```python
from build123d import *

# Parameters (mm, degrees)
ESBO_O1_W                = 6.6
ESBO_O1_H                = 2.5
RESSALTO_EXTRUS_O1_DEPTH = 20
ESBO_O2_R                = 1.5
CORTE_EXTRUS_O1_DEPTH    = 26
ESBO_O4_R                = 1.8
CORTE_EXTRUS_O2_DEPTH    = 16


with BuildPart() as part:
    # Esboço1 → Ressalto-extrusão1 (new body)
    with BuildSketch(Plane.XY):
        with BuildLine():
            Line((-12, 0), (-12, -7))
            Line((-12, -7), (-21, -7))
            Line((-21, -7), (-21, -10))
            Line((-21, -10), (54, -10))
            Line((54, -10), (54, -7))
            Line((54, -7), (45, -7))
            Line((45, -7), (45, 0))
            ThreePointArc((45, 0), (43.507140429, 5.796550698), (39.4, 10.150862032))
            ThreePointArc((39.4, 10.150862032), (38.373214893, 11.239439866), (38, 12.68857754))
            Line((38, 12.68857754), (38, 15.080826084))
            Line((38, 15.080826084), (28, 15.080826084))
            Line((28, 15.080826084), (28, 12.68857754))
            ThreePointArc((28, 12.68857754), (27.626785107, 11.239439866), (26.6, 10.150862032))
            ThreePointArc((26.6, 10.150862032), (22.492859571, 5.796550698), (21, 0))
            Line((21, 0), (21, -7))
            Line((21, -7), (12, -7))
            Line((12, -7), (12, 0))
            ThreePointArc((12, 0), (10.507140429, 5.796550698), (6.4, 10.150862032))
            ThreePointArc((6.4, 10.150862032), (5.373214893, 11.239439866), (5, 12.68857754))
            Line((5, 12.68857754), (5, 15.080826084))
            Line((5, 15.080826084), (-5, 15.080826084))
            Line((-5, 15.080826084), (-5, 12.68857754))
            ThreePointArc((-5, 12.68857754), (-5.373214893, 11.239439866), (-6.4, 10.150862032))
            ThreePointArc((-6.4, 10.150862032), (-10.507140429, 5.796550698), (-12, 0))
        make_face()
        with Locations((0, 10.080826084)):
            Rectangle(ESBO_O1_W, ESBO_O1_H, mode=Mode.SUBTRACT)
        with Locations((33, 10.080826084)):
            Rectangle(ESBO_O1_W, ESBO_O1_H, mode=Mode.SUBTRACT)
        with BuildLine():
            ThreePointArc((7.8, 0), (0, 7.8), (-7.8, 0))
            ThreePointArc((-7.8, 0), (0, -7.8), (7.8, 0))
        make_face(mode=Mode.SUBTRACT)
        with BuildLine():
            ThreePointArc((40.8, 0), (33, -7.8), (25.2, 0))
            ThreePointArc((25.2, 0), (33, 7.8), (40.8, 0))
        make_face(mode=Mode.SUBTRACT)
    extrude(amount=RESSALTO_EXTRUS_O1_DEPTH)

    # Esboço2 → Corte-extrusão1 (cut)
    with BuildSketch(Plane(origin=(0, -7, 0), x_dir=(1, 0, 0), z_dir=(0, 1, 0))):
        with Locations((-16.5, -4)):
            Circle(ESBO_O2_R)
        with Locations((-16.5, -16)):
            Circle(ESBO_O2_R)
        with Locations((49.5, -16)):
            Circle(ESBO_O2_R)
        with Locations((49.5, -4)):
            Circle(ESBO_O2_R)
        with Locations((16.5, -10)):
            Circle(ESBO_O2_R)
    extrude(amount=-CORTE_EXTRUS_O1_DEPTH, mode=Mode.SUBTRACT)

    # Esboço4 → Corte-extrusão2 (cut)
    with BuildSketch(Plane(origin=(0, 15.080826084, 0), x_dir=(1, 0, 0), z_dir=(0, 1, 0))):
        with Locations((0, -10)):
            Circle(ESBO_O4_R)
        with Locations((33, -10)):
            Circle(ESBO_O4_R)
    extrude(amount=-CORTE_EXTRUS_O2_DEPTH, mode=Mode.SUBTRACT)


solid = part.part
```
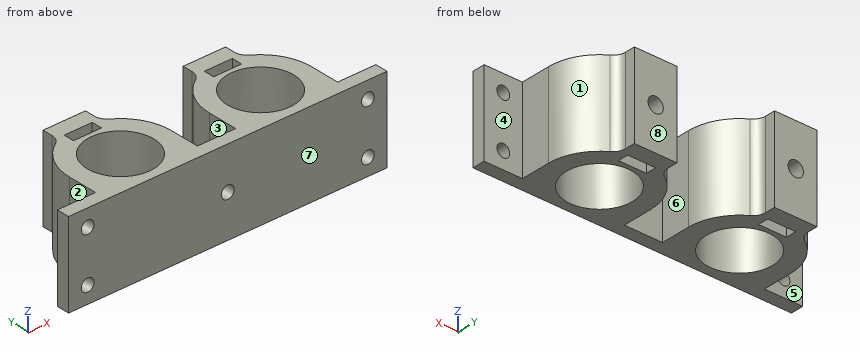
Verification items for the finished model (mm, model axes). Face numbers are marked on the shaded views. A direction names the side the tool comes from. Give positions to 0.01 mm unless a question says otherwise; leave off trailing zeros. Order: outer loops, then holes, each group sorted by start corner. A loop starts at its lowest first (then second) coordinate and runs counter-clockwise, first axis right, second up. Notation, with made-up numbers: (3.25, 48) - (15.25, 48) arc R34 cw to (15.25, 79) - close; hole circle Ø4 at (56.25, 89). An arc over 180 degrees is marked (long way). Answer as CSV lines item,"result". Start each with the question number.
Item 1: Access from +Z, -Z, +X, -X, +Y, -Y to the whole of each face (thin tool, end or side, straight path). Record for the marked faces 4, 5, 6, 7 and 8.
Item 2: Material ranges on L1, parallel to X at y = -9.2, z = 16; L2, parallel to X at y = -0.5, z = 17.75; L3, parallel to X at y = 9.75, z = 5.25, recorded low to high.
Item 3: Mould release check, pull along X, two halves, no side actions. Record for the marked faces 1, 2 and 3: released by +X, released by -X, zero draft, split by the parting line, or undercut.
Item 4: Section check D-D, the plane y = -6. Record the boundary of the cut face in (x, z).
Item 5: Section check B-B, the plane y = 1. Record the boundary of the cut face in (x, z), plus the area to 3 significant figures.
Item 6: Gauge pin test, flat ends, axial feed: pin 1 (8 mm diameter, centred on y = 4.5, z = 17, fed in from -X); pin 2 (1.2 mm diameter, centred on y = 14, z = 13, fed in from +X); pin 3 (4.5 mm diameter, centred on x = -18.5, z = 10.5, fed in from +Y); pin 4 (1.5 mm diameter, centred on x = 39, y = -4.5, fed in from -Z). Record the tip position at first contact, or that the pin passes through.
Item 7: Section check C-C, the plane x = 16.5. Record the boundary of the cut face in (y, z).
Item 8: Section check A-A, the plane x = 33. Record the boundary of the cut face in (y, z).
Filled in:
1,face 4,"+Z, -Z, +X, +Y"
1,face 5,"+Z, -Z, -X, +Y"
1,face 6,"+Z, -Z, +Y"
1,face 7,"+Z, -Z, +X, -X, -Y"
1,face 8,"+Z, -Z, +X, -X, +Y"
2,L1,"-21 to -18, -15 to 48, 51 to 54"
2,L2,"-12 to -7.78, 7.78 to 12, 21 to 25.22, 40.78 to 45"
2,L3,"-7 to -3.3, 3.3 to 7, 26 to 29.7, 36.3 to 40"
3,face 1,"released by +X"
3,face 2,"released by -X"
3,face 3,"undercut"
4,outline,"(-12, 0) - (-4.98, 0) - (-4.98, 20) - (-12, 20) - close; (4.98, 0) - (12, 0) - (12, 20) - (4.98, 20) - close; (21, 0) - (28.02, 0) - (28.02, 20) - (21, 20) - close; (37.98, 0) - (45, 0) - (45, 20) - (37.98, 20) - close"
5,outline,"(-11.96, 0) - (-7.74, 0) - (-7.74, 20) - (-11.96, 20) - close; (7.74, 0) - (11.96, 0) - (11.96, 20) - (7.74, 20) - close; (21.04, 0) - (25.26, 0) - (25.26, 20) - (21.04, 20) - close; (40.74, 0) - (44.96, 0) - (44.96, 20) - (40.74, 20) - close"
5,area,"338 mm^2"
6,pin 1,"x = -11.99"
6,pin 2,"x = 38"
6,pin 3,"y = -7"
6,pin 4,"z = 0"
7,outline,"(-10, 0) - (-7, 0) - (-7, 8.5) - (-10, 8.5) - close; (-10, 11.5) - (-7, 11.5) - (-7, 20) - (-10, 20) - close"
8,outline,"(-10, 0) - (-7.8, 0) - (-7.8, 20) - (-10, 20) - close; (7.8, 0) - (8.83, 0) - (8.83, 8.2) - (7.8, 8.2) - close; (7.8, 11.8) - (8.83, 11.8) - (8.83, 20) - (7.8, 20) - close; (11.33, 0) - (15.08, 0) - (15.08, 8.2) - (11.33, 8.2) - close; (11.33, 11.8) - (15.08, 11.8) - (15.08, 20) - (11.33, 20) - close"
